Can you work these out from the model? Positions are in its coordinate system, mm. Give positions to 0.01 mm unless a question says otherwise; leave off trailing zeros. Order: outer loops, then holes, each group sorted by start corner. A loop starts at its lowest first (then second) coordinate and runs counter-clockwise, first axis right, second up. Notation, with made-up numbers: M 57,-32.75 L 86,-32.75 A21 cw 86,-15.75 Z; hole C 84.5,-35.75 d2. An arc over 180 degrees is marked long. One line per question, with ' | ' between items. Start each with the question number.
1) Thinking about a two-plate mould opening in X: for faces 1 (the flat face through (1, 0, 15)), 2 (the cylindrical face through (-3, 5, 0)), 3 (the cylindrical face through (-94.432, 5.07, -1)), 4 (the cylindrical face through (94.432, 5.07, 1)), which applies, +X half, -X half, draft (parallel to the pull), parting line (faces both ways), or undercut?
2) If we section it at C-C, the plane y = 8: Please give me the cut outline in (x, z), plus the area to 3 significant figures.
3) If we section it at B-B, the plane x = 0: Please give me the cut outline in (y, z), plus the area to 3 significant figures.
4) If we section it at D-D, the plane z = -50.5: Please give me the cut outline in (x, y), plus the area to 3 significant figures.
5) I'm going to push flat-ended pins straight in: pin 1 Ø2 at (y, z) = (3, 28) entering from -X; pin 2 Ø1 at (x, z) = (48, 43.5) entering from -Y; pin 3 Ø1 at (y, z) = (8.5, -22) entering from +X; pin 4 Ø4 at (y, z) = (4.5, -24.5) entering from +X. Where does each tip first touch, or does it pass through?
6) If we section it at A-A, the plane z = 0: Please give me the cut outline in (x, y).
7) Please list where these lines run through material, in increasing order: line 1 along Z through (x, y) = (0, 3); line 2 along X through (y, z) = (4.5, -46); line 3 along X through (y, z) = (8.5, 47). Write a range as [from, to].
Autodesk Inventor part; units mm, degrees
ref_plane "YZ Plane" through (0, 0, 0) normal (1, 0, 0) x (0, 1, 0)
ref_plane "XZ Plane" through (0, 0, 0) normal (0, 1, 0) x (-1, 0, 0)
ref_plane "XY Plane" through (0, 0, 0) normal (0, 0, 1) x (1, 0, 0)
sketch "Sketch1" plane through (0, 0, 0) normal (0, 1, 0) x (-1, 0, 0)
  line L0 (70, 65.5) -> (-70, 65.5)
  line L1 (-70, 65.5) -> (-70, -65.5)
  line L2 (-70, -65.5) -> (70, -65.5)
  line L3 (70, -65.5) -> (70, 65.5)
  line L4 (70, 65.5) -> (-70, -65.5) construction
  line L5 (-70, 65.5) -> (70, -65.5) construction
  circle A0 centre (0, 0) radius 7.5
  dimension "d0" = 140
  dimension "d1" = 131
  dimension "d2" = 15
extrude "Extrusion1" add sketch "Sketch1" along normal blind 10
sketch "Sketch2" plane through (0, 10, 0) normal (0, 1, 0) x (1, 0, 0)
  circle A0 centre (0, 0) radius 7.5
  circle A1 centre (0, 0) radius 3
  dimension "d5" = 6
extrude "Extrusion2" add sketch "Sketch2" against normal blind 10
sketch "Sketch3" plane through (0, 10, 0) normal (0, 1, 0) x (1, 0, 0)
  line L0 (70, -65.5) -> (70, 65.5)
  line L1 (-70, 65.5) -> (-70, -65.5)
  arc A0 (70, -65.5) -> (70, 65.5) centre (-5.5629, 0) ccw
  arc A1 (-70, 65.5) -> (-70, -65.5) centre (5.5629, 0) ccw
  dimension "d10" = 100
  dimension "d11" = 100
extrude "Extrusion3" add sketch "Sketch3" against normal blind 10
properties part number "deska_pod_rameno"
Results found:
1) face 1: draft | face 2: undercut | face 3: -X half | face 4: +X half
2) outline: M -70,-65.5 L 70,-65.5 A100 ccw 70,65.5 L -70,65.5 A100 ccw Z; hole C 0,0 d6 | area: 22,700 mm²
3) outline: M 0,-65.5 L 10,-65.5 L 10,-3 L 0,-3 Z; M 0,3 L 10,3 L 10,65.5 L 0,65.5 Z | area: 1,250 mm²
4) outline: M -80.75,0 L 80.75,0 L 80.75,10 L -80.75,10 Z | area: 1,610 mm²
5) pin 1: stops at x = -90.72 | pin 2: stops at y = 0 | pin 3: stops at x = 92.1 | pin 4: stops at x = 91.87
6) outline: M -94.44,0 L -3,0 L -3,10 L -94.44,10 Z; M 3,0 L 94.44,0 L 94.44,10 L 3,10 Z
7) line 1: z = [-65.5, -3], [3, 65.5] | line 2: x = [-83.23, 83.23] | line 3: x = [-82.7, 82.7]
